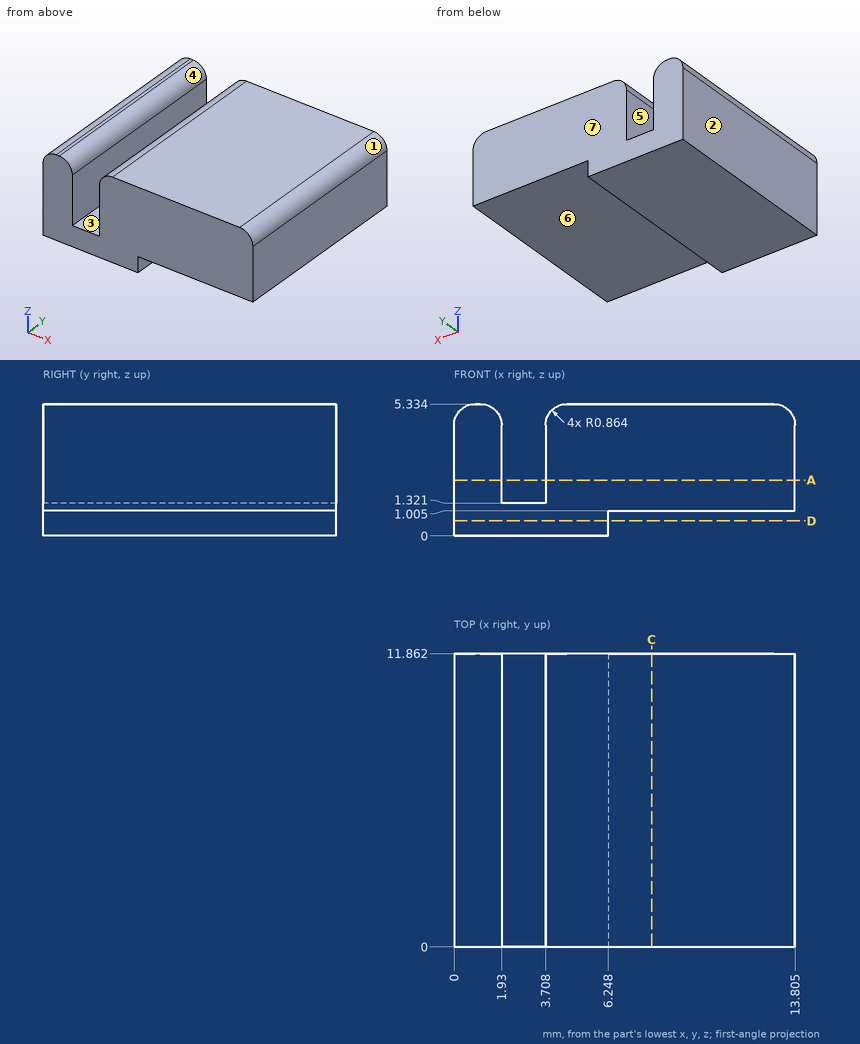
Study the drawing (mm; zero at the part's minimum x, y, z) and answer. A direction names the side the tool comes from. Round coordinates to 2 decimals unless told otherwise and drop trailing zeros. Write each loop counter-clockwise with the first axis right and the second up, starting at its lowest first coordinate (ties: lowest second). Pieces come first, ordered by that corner, then holes.
1) Straight lines are drawn through the part: line 1 (X direction, y = 3.75, z = 2.4) (1 decimal); line 2 (Z direction, x = 9.25, y = 3.25) (1 decimal); line 3 (Z direction, x = 4.5, y = 4.5). For each, find the intervals that lie inside material, in ascending order.
2) A cutting plane is placed at D-D (z = 0.6). Give the vertices of the cut face in (x, y).
3) A cutting plane is placed at A-A (z = 2.25). Give the vertices of the cut face in (x, y) (1 decimal), plus the area to 3 significant figures.
4) The mould has two halves that part along X. Classify the marked faces 1, 2, 3 and 4: pulls with the +X half, pulls with the -X half, needs draft (parallel to the pull), parting line crosses it, or undercut.
5) A tool of negligible diameter and unlimited length cuts with its end or side. For the marked faces 5, 6 and 7, from which of +Z, -Z, +X, -X, +Y, -Y can it reach the whole face along a straight path? Write none if from no direction.
6) A cutting plane is placed at C-C (x = 8). Give the vertices of the cut face in (y, z) (1 decimal).
7) Given pin 1 Ø4 at (x, y) = (11, 8.5) entering from -Z (1 decimal); pin 2 Ø0.5 at (x, y) = (3, 7.5) entering from +Z; pin 3 Ø0.5 at (y, z) = (8, 0.5) entering from +X, each flat-ended and moving along its own axis, determine where each tip first touches the part or whether it passes through.
Completed:
1. line 1: x = 0 to 1.9, 3.7 to 13.8
1. line 2: z = 1 to 5.3
1. line 3: z = 0 to 5.33
2. outline: (0, 0) - (6.25, 0) - (6.25, 11.86) - (0, 11.86) - close
3. outline: (0, 0) - (1.9, 0) - (1.9, 11.9) - (0, 11.9) - close; (3.7, 0) - (13.8, 0) - (13.8, 11.9) - (3.7, 11.9) - close
3. area: 143 mm2
4. face 1: pulls with the +X half
4. face 2: pulls with the -X half
4. face 3: undercut
4. face 4: undercut
5. face 5: +Z, +Y, -Y
5. face 6: -Z, +X, +Y, -Y
5. face 7: +Z, -Z, +X, -X, +Y
6. outline: (0, 1) - (11.9, 1) - (11.9, 5.3) - (0, 5.3) - close
7. pin 1: stops at z = 1
7. pin 2: stops at z = 1.32
7. pin 3: stops at x = 6.25
